```python
from build123d import *

# Parameters (mm, degrees)
SKETCH1_W           = 12.7
SKETCH1_H           = 76.2
SKETCH1_W_2         = 5.08
SKETCH1_W_3         = 9.652
SKETCH1_H_2         = 3.175
BOSS_EXTRUDE1_DEPTH = 1.5875


with BuildPart() as part:
    # Sketch1 → Boss-Extrude1 (new body)
    with BuildSketch(Plane(origin=(0, 0, 0), x_dir=(1, 0, 0), z_dir=(0, 1, 0))):
        with Locations((11.43, 38.1)):
            Rectangle(SKETCH1_W, SKETCH1_H)
        with Locations((2.54, 38.1)):
            Rectangle(SKETCH1_W_2, SKETCH1_H)
        with Locations((22.606, 38.1)):
            Rectangle(SKETCH1_W_3, SKETCH1_H)
        with Locations((11.43, -1.5875)):
            Rectangle(SKETCH1_W, SKETCH1_H_2)
        with Locations((11.43, 77.7875)):
            Rectangle(SKETCH1_W, SKETCH1_H_2)
    extrude(amount=BOSS_EXTRUDE1_DEPTH)


solid = part.part
```
Could you check a few things on this model? Use its own coordinates, in mm. A direction names the side the tool comes from. Round coordinates to 2 decimals unless told otherwise and drop trailing zeros. Write each loop counter-clockwise with the first axis right and the second up, starting at its lowest first coordinate (ties: lowest second). Pieces come first, ordered by that corner, then holes. Notation, with made-up numbers: M 61.25,52 L 87.25,52 A16 cw 87.25,79 Z; hole C 82.25,-14 d2. An arc over 180 degrees is marked long. Write each question's results on one line, items separated by ' | '. Start each with the question number.
1. I'm going to push flat-ended pins straight in: pin 1 Ø0.5 at (y, z) = (1, -78) entering from -X; pin 2 Ø0.5 at (x, y) = (3, 1) entering from -Z; pin 3 Ø0.8 at (x, y) = (2, 1) entering from +Z. Where does each tip first touch, or does it pass through?
2. I need wall thicknesses on L1, parallel to Z at x = 20.75, y = 0.7. Which ranges of the line are inside material? Lowest first, please. Write a range as from..to.
3. Imagine slicing it at A-A on y = 0.3. List the corners of the cut face in (x, z) for me (3 decimals).
4. On a 3-axis mill with a long thin cutter (end or side, diameter ignored), from which of +Z, -Z, +X, -X, +Y, -Y can I reach the whole of each face in a straight line? I mean faces 1 (the face through (23, 1, -76.2)), 2 (the face through (5.08, 1, 2)), 3 (the face through (3, 1, -76.2)). Say none if no direction works.
Result sheet:
1) pin 1: stops at x = 5.08 | pin 2: stops at z = -76.2 | pin 3: stops at z = 0
2) L1: z = -76.2..0
3) outline: M 0,-76.2 L 5.08,-76.2 L 5.08,-79.375 L 17.78,-79.375 L 17.78,-76.2 L 27.432,-76.2 L 27.432,0 L 17.78,0 L 17.78,3.175 L 5.08,3.175 L 5.08,0 L 0,0 Z
4) face 1: -Z, +X, +Y, -Y | face 2: +Z, -X, +Y, -Y | face 3: -Z, -X, +Y, -Y
